from build123d import *

# Parameters (mm, degrees)
F0_W     = 254
F0_H     = 254
F1_DEPTH = 254
F4_T     = -25.4
F7_W     = 101.6
F7_H     = 76.2
F5_DEPTH = 203.2


with BuildPart() as f1:
    # F0 (on Right) → F1 (new body)
    with BuildSketch(Plane.YZ):
        with Locations((-127, -127)):
            Rectangle(F0_W, F0_H)
    extrude(amount=F1_DEPTH)

    # F2 (on face) → F3 (revolve, cut)
    with BuildSketch(Plane.YZ.offset(254)):
        with BuildLine():
            Line((-200.374284178, 0), (-53.625715822, 0))
            ThreePointArc((-53.625715822, 0), (-127, 19.6723749676), (-200.374284178, 0))
        make_face()
        with BuildLine():
            Line((0, -127), (0, -53.625715822))
            ThreePointArc((0, -53.625715822), (-23.2869690477, -23.2869690477), (-53.625715822, 0))
            Line((-53.625715822, 0), (-200.374284178, 0))
            ThreePointArc((-200.374284178, 0), (-230.7130309523, -23.2869690477), (-254, -53.625715822))
            Line((-254, -53.625715822), (-254, -127))
            Line((-254, -127), (0, -127))
        make_face()
        with BuildLine():
            Line((0, -127), (19.6723749676, -127))
            ThreePointArc((19.6723749676, -127), (14.6689401378, -89.0171488843), (0, -53.625715822))
            Line((0, -53.625715822), (0, -127))
        make_face()
        with BuildLine():
            Line((-273.6723749676, -127), (-254, -127))
            Line((-254, -127), (-254, -53.625715822))
            ThreePointArc((-254, -53.625715822), (-268.6689401378, -89.0171488843), (-273.6723749676, -127))
        make_face()
    revolve(axis=Axis((254, -127, -127), (0, -1, 0)), mode=Mode.SUBTRACT)

    # F4
    f4_openings = [f1.faces().sort_by_distance(p)[0] for p in [
        (0, -127, -127),
    ]]
    offset(amount=F4_T, openings=f4_openings)

    # F7 (on Right) → F5 (join)
    with BuildSketch(Plane.YZ):
        with Locations((-50.8, 38.1)):
            Rectangle(F7_W, F7_H)
    extrude(amount=F5_DEPTH)


solid = f1.part
Work out the finished part from the listing and answer in its coordinate system (mm). A direction names the side the tool comes from. Give positions to 0.01 mm unless a question says otherwise; leave off trailing zeros. Write each loop counter-clockwise with the first axis right and the second up, starting at its lowest first coordinate (ties: lowest second). Pieces come first, ordered by that corner, then holes. Notation, with made-up numbers: (81, 48) - (128, 48) arc R17 cw to (128, 75) - close; hole circle Ø9 at (55, 33). An arc over 180 degrees is marked (long way). One line per item, written item: value. Start each with the question number.
1. Find section B-B (x = 95). Write down the section's boundary in (y, z), then the cut area to 3 significant figures.
2. For a pull along Z with two mould halves and no side action, classify faces 4 (the flat face through (61, -128, -228.6)), 5 (the flat face through (97, -179, 0)), 6 (the flat face through (97, 0, -91)) as +Z half, -Z half, draft (parallel to the pull), parting line (faces both ways), or undercut.
3. For faces 1 (the flat face through (203.2, -52, 39)), 2 (the flat face through (61, -128, -25.4)), 3 (the flat face through (196, -91, 0)), determine the directions among +Z, -Z, +X, -X, +Y, -Y from which every point of the face is accessible in a straight line to the end or side of a thin tool.
4. Consider probe 1 along Z at (x, y) = (88, -67.5); probe 2 along Y at (x, z) = (106, -70); probe 3 along Z at (x, y) = (55.5, -158.5). Determine where each line is inside the solid, lowest interval first.
5. Find section A-A (x = 21). Write down the section's boundary in (y, z).
6. Find section D-D (x = 208). Write down the section's boundary in (y, z), then the cut area to 3 significant figures.
7. Find section C-C (y = -180). Write down the section's boundary in (x, z), then the cut area to 3 significant figures.
8. Given pin 1 (23 mm diameter, centred on y = -41, z = 33, fed in from +X); pin 2 (12 mm diameter, centred on x = 72, y = -156, fed in from +Z); pin 3 (12 mm diameter, centred on y = -77.5, z = -89.5, fed in from -X), each flat-ended and moving along its own axis, determine where each tip first touches the part or whether it passes through.
Geometry results:
1. outline: (-254, -254) - (0, -254) - (0, 76.2) - (-101.6, 76.2) - (-101.6, 0) - (-254, 0) - close; circle Ø131.57 at (-127, -127); hole (-228.6, -228.6) - (-25.4, -228.6) - (-25.4, -25.4) - (-228.6, -25.4) - close
1. area: 44,600 mm2
2. face 4: undercut
2. face 5: +Z half
2. face 6: draft
3. face 1: +Z, +X, +Y, -Y
3. face 2: -X
3. face 3: -Z, +X
4. probe 1: -254 to -228.6, -25.4 to 76.2
4. probe 2: -254 to -228.6, -193.75 to -60.25, -25.4 to 0
4. probe 3: -254 to -228.6, -25.4 to 0
5. outline: (-254, -254) - (0, -254) - (0, 76.2) - (-101.6, 76.2) - (-101.6, 0) - (-254, 0) - close; hole (-228.6, -228.6) - (-25.4, -228.6) - (-25.4, -25.4) - (-228.6, -25.4) - close
6. outline: (-254, -254) - (-184.16, -254) arc R139.27 cw to (-254, -184.16) - close; (-254, -69.84) arc R139.27 cw to (-184.16, 0) - (-254, 0) - close; (-69.84, -254) - (0, -254) - (0, -184.16) arc R139.27 cw to start; (-69.84, 0) arc R139.27 cw to (0, -69.84) - (0, 0) - close
6. area: 7,360 mm2
7. outline: (0, -254) - (203.26, -254) arc R136.76 cw to (203.26, 0) - (0, 0) - (0, -25.4) - (125.64, -25.4) arc R163.71 ccw to (125.64, -228.6) - (0, -228.6) - close
7. area: 15,200 mm2
8. pin 1: x = 203.2
8. pin 2: z = 0
8. pin 3: x = 91.33
